Work out the finished part from the listing and answer in its coordinate system (mm). Coordinates: 2 decimals unless noted, no trailing zeros. Order: outer loops, then holes, each group sorted by start corner. A loop starts at its lowest first (then second) coordinate and runs counter-clockwise, first axis right, second up. Notation, with made-up numbers: M 20,-19.75 L 28,-19.75 A23 ccw 28,9.25 Z; hole C 30.25,-22.75 d10. An arc over 180 degrees is marked long. Use a Markdown table: item, result. Add a question column.
from build123d import *

# Parameters (mm, degrees)
ESQUISSE1_W               = 203.2
ESQUISSE1_H               = 203.2
BOSS_EXTRU_1_DEPTH        = 6.35
ESQUISSE2_R               = 3.925
ENL_V_MAT_EXTRU_1_DEPTH   = 144.824345992
ENL_V_MAT_EXTRU_2_DEPTH   = 144.824345992
ENL_V_MAT_EXTRU_5_DEPTH   = 144.824345992
ENL_V_MAT_EXTRU_6_DEPTH   = 144.824345992
ENL_V_MAT_EXTRU_7_DEPTH   = 144.824345992
ENL_V_MAT_EXTRU_8_DEPTH   = 144.824345992
ENL_V_MAT_EXTRU_9_DEPTH   = 144.824345992
ESQUISSE11_R              = 2.5
ENL_V_MAT_EXTRU_10_DEPTH  = 144.824345992
ESQUISSE12_R              = 4
ENL_V_MAT_EXTRU_11_DEPTH  = 144.824345992
ESQUISSE13_R              = 2.5
ENL_V_MAT_EXTRU_12_DEPTH  = 144.824345992
SYM_TRIE2_COPY_1_SKETCH_R = 2.5
SYM_TRIE2_COPY_1_DEPTH    = 144.824345992
CONG_3_R                  = 4
ENL_V_MAT_EXTRU_13_DEPTH  = 144.824345992
ESQUISSE15_R              = 2.6
ENL_V_MAT_EXTRU_14_DEPTH  = 144.824345992
ENL_V_MAT_EXTRU_15_DEPTH  = 144.824345992


with BuildPart() as part:
    # Esquisse1 → Boss.-Extru.1 (new body)
    with BuildSketch(Plane(origin=(0, 0, 0), x_dir=(1, 0, 0), z_dir=(0, 1, 0))):
        Rectangle(ESQUISSE1_W, ESQUISSE1_H)
    extrude(amount=BOSS_EXTRU_1_DEPTH)

    # Esquisse2 → Enlèv. mat.-Extru.1 (cut, through all)
    with BuildSketch(Plane(origin=(0, 6.35, 0), x_dir=(1, 0, 0), z_dir=(0, 1, 0))):
        with Locations(Location((-75, 65, 0), (0, 0, 270))):
            Circle(ESQUISSE2_R)
        with Locations(Location((75, 65, 0), (0, 0, 270))):
            Circle(ESQUISSE2_R)
        with Locations(Location((0, -65, 0), (0, 0, 270))):
            Circle(ESQUISSE2_R)
    extrude(amount=-ENL_V_MAT_EXTRU_1_DEPTH, mode=Mode.SUBTRACT)

    # Esquisse3 → Enlèv. mat.-Extru.2 (cut, through all)
    with BuildSketch(Plane(origin=(0, 6.35, 0), x_dir=(1, 0, 0), z_dir=(0, 1, 0))):
        Polygon((-16.978069991, 86.15), (-21.15, 81.978069991), (-21.15, 48.021930009), (-16.978069991, 43.85), (16.978069991, 43.85), (21.15, 48.021930009), (21.15, 81.978069991), (16.978069991, 86.15), align=None)
    extrude(amount=-ENL_V_MAT_EXTRU_2_DEPTH, mode=Mode.SUBTRACT)

    # Esquisse5 → Enlèv. mat.-Extru.5 (cut, through all)
    with BuildSketch(Plane(origin=(0, 6.35, 0), x_dir=(1, 0, 0), z_dir=(0, 1, 0))):
        Polygon((-31.3966679, 49.85), (-33.64833395, 45.95), (-38.15166605, 45.95), (-40.4033321, 49.85), (-38.15166605, 53.75), (-33.64833395, 53.75), align=None)
    extrude(amount=-ENL_V_MAT_EXTRU_5_DEPTH, mode=Mode.SUBTRACT)

    # Esquisse7 → Enlèv. mat.-Extru.6 (cut, through all)
    with BuildSketch(Plane(origin=(0, 6.35, 0), x_dir=(1, 0, 0), z_dir=(0, 1, 0))):
        Polygon((-33.64833395, 75.95), (-38.15166605, 75.95), (-40.4033321, 79.85), (-38.15166605, 83.75), (-33.64833395, 83.75), (-31.3966679, 79.85), align=None)
    extrude(amount=-ENL_V_MAT_EXTRU_6_DEPTH, mode=Mode.SUBTRACT)

    # Esquisse8 → Enlèv. mat.-Extru.7 (cut, through all)
    with BuildSketch(Plane(origin=(0, 6.35, 0), x_dir=(1, 0, 0), z_dir=(0, 1, 0))):
        Polygon((37.85166605, 45.95), (33.34833395, 45.95), (31.0966679, 49.85), (33.34833395, 53.75), (37.85166605, 53.75), (40.1033321, 49.85), align=None)
    extrude(amount=-ENL_V_MAT_EXTRU_7_DEPTH, mode=Mode.SUBTRACT)

    # Esquisse9 → Enlèv. mat.-Extru.8 (cut, through all)
    with BuildSketch(Plane(origin=(0, 6.35, 0), x_dir=(1, 0, 0), z_dir=(0, 1, 0))):
        Polygon((37.85166605, 75.95), (33.34833395, 75.95), (31.0966679, 79.85), (33.34833395, 83.75), (37.85166605, 83.75), (40.1033321, 79.85), align=None)
    extrude(amount=-ENL_V_MAT_EXTRU_8_DEPTH, mode=Mode.SUBTRACT)

    # Esquisse10 → Enlèv. mat.-Extru.9 (cut, through all)
    with BuildSketch(Plane(origin=(0, 6.35, 0), x_dir=(1, 0, 0), z_dir=(0, 1, 0))):
        Polygon((-11.085125168, -56), (-13.336791218, -52.1), (-17.840123318, -52.1), (-20.091789368, -56), (-17.840123318, -59.9), (-13.336791218, -59.9), align=None)
        Polygon((11.085125168, -56), (13.336791218, -59.9), (17.840123318, -59.9), (20.091789368, -56), (17.840123318, -52.1), (13.336791218, -52.1), align=None)
        Polygon((-4.5033321, -83), (-2.25166605, -86.9), (2.25166605, -86.9), (4.5033321, -83), (2.25166605, -79.1), (-2.25166605, -79.1), align=None)
        Polygon((-63.916340686, 55.999154304), (-61.664674636, 52.099154304), (-57.161342537, 52.099154304), (-54.909676487, 55.999154304), (-57.161342537, 59.899154304), (-61.664674636, 59.899154304), align=None)
        Polygon((-95.093255222, 55.999154304), (-92.841589173, 52.099154304), (-88.338257073, 52.099154304), (-86.086591023, 55.999154304), (-88.338257073, 59.899154304), (-92.841589173, 59.899154304), align=None)
        Polygon((-79.504797954, 82.999154304), (-77.253131904, 79.099154304), (-72.749799805, 79.099154304), (-70.498133755, 82.999154304), (-72.749799805, 86.899154304), (-77.253131904, 86.899154304), align=None)
        Polygon((54.908210632, 56), (57.159876682, 52.1), (61.663208782, 52.1), (63.914874832, 56), (61.663208782, 59.9), (57.159876682, 59.9), align=None)
        Polygon((95.091789368, 56), (92.840123318, 59.9), (88.336791218, 59.9), (86.085125168, 56), (88.336791218, 52.1), (92.840123318, 52.1), align=None)
        Polygon((70.4966679, 83), (72.74833395, 79.1), (77.25166605, 79.1), (79.5033321, 83), (77.25166605, 86.9), (72.74833395, 86.9), align=None)
    extrude(amount=-ENL_V_MAT_EXTRU_9_DEPTH, mode=Mode.SUBTRACT)

    # Esquisse11 → Enlèv. mat.-Extru.10 (cut, through all)
    with BuildSketch(Plane(origin=(0, 6.35, 0), x_dir=(1, 0, 0), z_dir=(0, 1, 0))):
        with Locations(Location((93.6, 93.6, 0), (0, 0, 270))):
            Circle(ESQUISSE11_R)
        with Locations(Location((-93.6, 93.6, 0), (0, 0, 270))):
            Circle(ESQUISSE11_R)
        with Locations(Location((-93.6, -93.6, 0), (0, 0, 270))):
            Circle(ESQUISSE11_R)
        with Locations(Location((93.6, -93.6, 0), (0, 0, 270))):
            Circle(ESQUISSE11_R)
    extrude(amount=-ENL_V_MAT_EXTRU_10_DEPTH, mode=Mode.SUBTRACT)

    # Esquisse12 → Enlèv. mat.-Extru.11 (cut, through all)
    with BuildSketch(Plane(origin=(0, 6.35, 0), x_dir=(1, 0, 0), z_dir=(0, 1, 0))):
        with Locations(Location((0, 10.325, 0), (0, 0, 270))):
            Circle(ESQUISSE12_R)
    extrude(amount=-ENL_V_MAT_EXTRU_11_DEPTH, mode=Mode.SUBTRACT)

    # Esquisse13 → Enlèv. mat.-Extru.12 (cut, through all)
    with BuildSketch(Plane.XZ):
        with Locations(Location((56, -85, 0), (0, 0, 270))):
            Circle(ESQUISSE13_R)
        with Locations(Location((82, 0, 0), (0, 0, 270))):
            Circle(ESQUISSE13_R)
    enl_v_mat_extru_12 = extrude(amount=-ENL_V_MAT_EXTRU_12_DEPTH, mode=Mode.SUBTRACT)

    # Symétrie1: Enlèv. mat.-Extru.12 across plane
    add(enl_v_mat_extru_12.mirror(Plane.XY), mode=Mode.SUBTRACT)

    # Symétrie2: Enlèv. mat.-Extru.12 across plane
    add(enl_v_mat_extru_12.mirror(Plane(origin=(0, 0, 0), x_dir=(0, 0, 1), z_dir=(1, 0, 0))), mode=Mode.SUBTRACT)

    # Symétrie2 copy 1 sketch → Symétrie2 copy 1 (cut, through all)
    with BuildSketch(Plane(origin=(0, 0, 0), x_dir=(-1, 0, 0), z_dir=(0, -1, 0))):
        with Locations(Location((56, -85, 0), (0, 0, 270))):
            Circle(SYM_TRIE2_COPY_1_SKETCH_R)
        with Locations(Location((82, 0, 0), (0, 0, 270))):
            Circle(SYM_TRIE2_COPY_1_SKETCH_R)
    extrude(amount=-SYM_TRIE2_COPY_1_DEPTH, mode=Mode.SUBTRACT)

    # Congé3
    cong_3_edges = [part.edges().sort_by_distance(p)[0] for p in [
        (101.6, 3.175, 101.6),
        (-101.6, 3.175, 101.6),
        (-101.6, 3.175, -101.6),
        (101.6, 3.175, -101.6),
    ]]
    fillet(cong_3_edges, radius=CONG_3_R)

    # Esquisse14 → Enlèv. mat.-Extru.13 (cut, through all)
    with BuildSketch(Plane(origin=(0, 6.35, 0), x_dir=(1, 0, 0), z_dir=(0, 1, 0))):
        Polygon((16.978069991, -42.150000003), (-16.978069991, -42.150000003), (-21.15, -37.978069994), (-21.15, -4.021930012), (-16.978069991, 0.149999997), (16.978069991, 0.149999997), (21.15, -4.021930012), (21.15, -37.978069994), align=None)
    extrude(amount=-ENL_V_MAT_EXTRU_13_DEPTH, mode=Mode.SUBTRACT)

    # Esquisse15 → Enlèv. mat.-Extru.14 (cut, through all)
    with BuildSketch(Plane(origin=(0, 6.35, 0), x_dir=(1, 0, 0), z_dir=(0, 1, 0))):
        with Locations(Location((35.6, -36.15, 0), (0, 0, 270))):
            Circle(ESQUISSE15_R)
        with Locations(Location((35.6, -6.15, 0), (0, 0, 270))):
            Circle(ESQUISSE15_R)
        with Locations(Location((-35.9, -36.15, 0), (0, 0, 270))):
            Circle(ESQUISSE15_R)
        with Locations(Location((-35.9, -6.15, 0), (0, 0, 270))):
            Circle(ESQUISSE15_R)
    extrude(amount=-ENL_V_MAT_EXTRU_14_DEPTH, mode=Mode.SUBTRACT)

    # Esquisse16 → Enlèv. mat.-Extru.15 (cut, through all)
    with BuildSketch(Plane(origin=(0, 6.35, 0), x_dir=(1, 0, 0), z_dir=(0, 1, 0))):
        Polygon((31.0966679, -36.15), (33.34833395, -40.05), (37.85166605, -40.05), (40.1033321, -36.15), (37.85166605, -32.25), (33.34833395, -32.25), align=None)
        Polygon((31.0966679, -6.15), (33.34833395, -10.05), (37.85166605, -10.05), (40.1033321, -6.15), (37.85166605, -2.25), (33.34833395, -2.25), align=None)
        Polygon((-40.4033321, -6.15), (-38.15166605, -10.05), (-33.64833395, -10.05), (-31.3966679, -6.15), (-33.64833395, -2.25), (-38.15166605, -2.25), align=None)
        Polygon((-40.4033321, -36.15), (-38.15166605, -40.05), (-33.64833395, -40.05), (-31.3966679, -36.15), (-33.64833395, -32.25), (-38.15166605, -32.25), align=None)
    extrude(amount=-ENL_V_MAT_EXTRU_15_DEPTH, mode=Mode.SUBTRACT)


solid = part.part
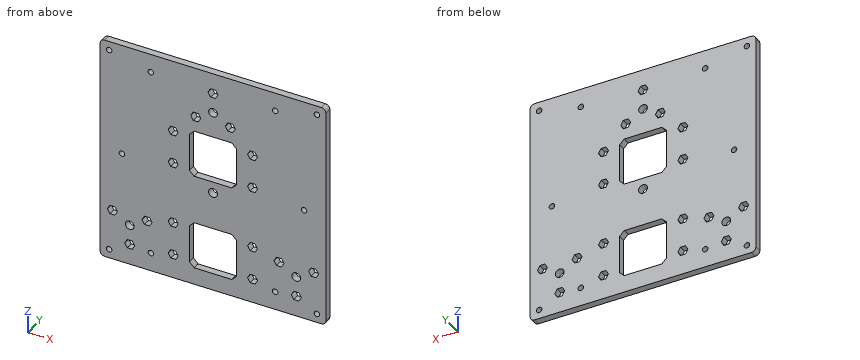
(1) A cutting plane is placed at C-C on z = -93.6. Write down the section's boundary in (x, y).
(2) A cutting plane is placed at D-D on y = 5.25. Count the separate pieces of the cut face and the enclosed holes in it, plus the area to 3 significant figures.
(3) A cutting plane is placed at A-A on z = 16.5. Write down the section's boundary in (x, y).
(4) A cutting plane is placed at B-B on x = 82. Write down the section's boundary in (y, z), plus the area to 3 significant figures.
(5) Straight lines are drawn through the part: line 1 (X direction, y = 3, z = -65) (3 decimals); line 2 (X direction, y = 4.5, z = 17.5); line 3 (X direction, y = 3.5, z = 85). For each, find the intervals that lie inside material, in ascending order.
From the geometry:
| question | item | result |
|---|---|---|
| 1 | outline | M -101.6,0 L -96.1,0 L -96.1,6.35 L -101.6,6.35 Z; M -91.1,0 L 91.1,0 L 91.1,6.35 L -91.1,6.35 Z; M 96.1,0 L 101.6,0 L 101.6,6.35 L 96.1,6.35 Z |
| 2 | separate pieces | 1 |
| 2 | enclosed holes | 33 |
| 2 | area | 36,500 mm2 |
| 3 | outline | M -101.6,0 L -21.15,0 L -21.15,6.35 L -101.6,6.35 Z; M 21.15,0 L 101.6,0 L 101.6,6.35 L 21.15,6.35 Z |
| 4 | outline | M 0,-101.6 L 6.35,-101.6 L 6.35,-2.5 L 0,-2.5 Z; M 0,2.5 L 6.35,2.5 L 6.35,101.6 L 0,101.6 Z |
| 4 | area | 1,260 mm2 |
| 5 | line 1 | x = -101.6 to -78.925, -71.075 to -21.15, 21.15 to 71.075, 78.925 to 101.6 |
| 5 | line 2 | x = -101.6 to -21.15, 21.15 to 101.6 |
| 5 | line 3 | x = -101.6 to -58.5, -53.5 to -3.35, 3.35 to 53.5, 58.5 to 101.6 |
